Study the drawing (mm; zero at the part's minimum x, y, z) and answer. Round coordinates to 2 decimals unless told otherwise and drop trailing zeros. Write each loop counter-clockwise with the first axis right and the second up, starting at its lowest first coordinate (ties: lowest second). Pieces come first, ordered by that corner, then holes. Notation, with made-up numbers: (33.5, 13.25) - (66.5, 13.25) arc R21 ccw to (66.5, 22.25) - close; hole circle Ø4 at (88, 42). An arc over 180 degrees is marked (long way). Use one line per item in the form item = value. Start each with the question number.
1) The part is cut by section A-A, the plane z = 1.7. Give the vertices of the cut face in (x, y), plus the area to 3 significant figures.
2) The part is cut by section C-C, the plane y = 5. Give the vertices of the cut face in (x, z), plus the area to 3 significant figures.
3) Consider line 1 along Y through (x, z) = (97, 1.85) (1 decimal); line 2 along Y through (x, z) = (5.5, 0.45) (1 decimal). Determine where each line is inside the solid, lowest interval first. Write a range as from..to.
4) The part is cut by section B-B, the plane y = 49.5. Give the vertices of the cut face in (x, z), plus the area to 3 significant figures.
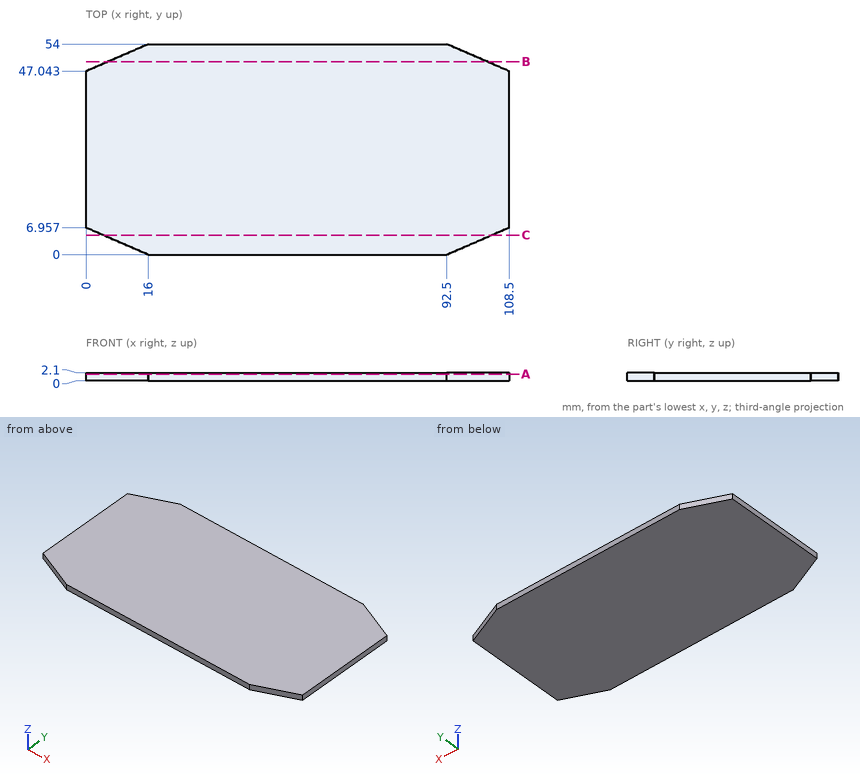
Geometry results:
q1.outline = (0, 6.96) - (16, 0) - (92.5, 0) - (108.5, 6.96) - (108.5, 47.04) - (92.5, 54) - (16, 54) - (0, 47.04) - close
q1.area = 5,640 mm2
q2.outline = (4.5, 0) - (104, 0) - (104, 2.1) - (4.5, 2.1) - close
q2.area = 209 mm2
q3.line_1 = 2..52
q3.line_2 = 4.6..49.4
q4.outline = (5.65, 0) - (102.85, 0) - (102.85, 2.1) - (5.65, 2.1) - close
q4.area = 204 mm2
